The model under review builds one solid part; all positions refer to its coordinate system, in mm. A direction names the side the tool comes from. Round coordinates to 2 decimals unless told otherwise and drop trailing zeros. Loops run counter-clockwise (first coordinate to the right, second up) from the corner with the lowest first, then second, coordinate; pieces in that order, holes last. Notation, with made-up numbers: (83.25, 59.5) -> (126.25, 59.5) arc R9 ccw to (126.25, 69.5) -> close; hole circle Ø8 at (-30, -28). An arc over 180 degrees is marked (long way). Write each question's results on one line, items separated by ' | '. Start each with the question number.
Item 1: Tool access review of faces 1 (the cylindrical face through (16, -2, 0)), 2 (the cylindrical face through (16.93, 5.635, 5.679)), 3 (the cylindrical face through (9, -1.08, -4.88)), 4 (the cylindrical face through (166, -6, 0)), 5 (the cylindrical face through (150.257, 2.731, 1.111)): name each direction out of +Z, -Z, +X, -X, +Y, -Y from which nothing blocks a thin tool from reaching the whole face with its end or side.
Item 2: Clearance check with flat-ended pins moving along their axes: pin 1 Ø3 at (x, y) = (160, 0) entering from -Z; pin 2 Ø3 at (x, y) = (90, -1.5) entering from +Z; pin 3 Ø2 at (x, y) = (106.5, -2) entering from -Z; pin 4 Ø7 at (x, y) = (166.5, -1.5) entering from -Z. State where each tip first meets the part, or that it passes through.
Item 3: Mouldability with a two-part tool opening along X and no side actions: class faces 6 (the flat face through (156.5, -0.1, 4)), 7 (the cylindrical face through (17.38, 3.97, 1.97)) as pulls with the +X half, pulls with the -X half, needs draft (parallel to the pull), parting line crosses it, or undercut.
Item 4: We need section A-A (x = 45). Give the boundary of the cut face in (y, z).
Item 5: For L1, parallel to Z at x = 152, y = 1.5; L2, parallel to X at y = 2.75, z = 4.5; L3, parallel to X at y = -0.25, z = -1.75, list the stretches that pass through material, from the lowest coordinate up. Write a range as from..to.
Autodesk Inventor part; units mm, degrees
ref_plane "FDT_FRONT_XY" through (12, 0, 0) normal (1, 0, 0) x (0, 0, -1)
ref_plane "FDT_FRONT_YZ" through (12, 0, 0) normal (0, 0, -1) x (0, 1, 0)
ref_plane "FDT_FRONT_ZX" through (12, 0, 0) normal (0, 1, 0) x (1, 0, 0)
sketch "Sketch_1" plane through (0, 0, 0) normal (0, 0, 1) x (1, 0, 0)
  line L0 (12, 0) -> (0, 0)
  line L1 (0, 0) -> (0, 5.15)
  line L2 (0, 5.15) -> (0.85, 6)
  line L3 (0.85, 6) -> (7.35, 6)
  line L4 (7.35, 6) -> (8.1743, 5.1757)
  arc A0 (8.1743, 5.1757) -> (8.5985, 5) centre (8.5985, 5.6) ccw
  line L5 (8.5985, 5) -> (9.4, 5)
  arc A1 (9.4, 5) -> (10, 5.6) centre (9.4, 5.6) ccw
  line L6 (10, 5.6) -> (10, 6)
  line L7 (10, 6) -> (12, 6)
  line L8 (12, 6) -> (12, 0)
  line L9 (12, 0) -> (0, 0)
revolve "Revolution1" add sketch "Sketch_1" angle 360 about axis through (12, 0, 0) along (1, 0, 0)
thread "Thread1"
sketch "Sketch_2" plane through (12, 0, 0) normal (1, 0, 0) x (0, 0, -1)
  arc A0 (-7, -3.873) -> (-3.873, -7) centre (0, 0) ccw
  line L0 (-3.873, -7) -> (3.873, -7)
  arc A1 (3.873, -7) -> (7, -3.873) centre (0, 0) ccw
  line L1 (7, -3.873) -> (7, 3.873)
  arc A2 (7, 3.873) -> (3.873, 7) centre (0, 0) ccw
  line L2 (3.873, 7) -> (-3.873, 7)
  arc A3 (-3.873, 7) -> (-7, 3.873) centre (0, 0) ccw
  line L3 (-7, 3.873) -> (-7, -3.873)
extrude "Extrusion1" add sketch "Sketch_2" along normal blind 10
sketch "Sketch_3" plane through (0, 0, 0) normal (0, 0, 1) x (1, 0, 0)
  line L0 (148, 0) -> (22, 0)
  line L1 (22, 0) -> (22, 4.65)
  line L2 (22, 4.65) -> (148, 4.65)
  line L3 (148, 4.65) -> (148, 0)
  line L4 (148, 0) -> (22, 0)
revolve "Revolution2" add sketch "Sketch_3" angle 360 about axis through (148, 0, 0) along (1, 0, 0)
sketch "Sketch_16" plane through (148, 0, 0) normal (1, 0, 0) x (0, 0, -1)
  line L0 (-7, -7) -> (7, -7)
  line L1 (7, -7) -> (7, 7)
  line L2 (7, 7) -> (-7, 7)
  line L3 (-7, 7) -> (-7, -7)
extrude "Extrusion2" add sketch "Sketch_16" along normal blind 10
sketch "Sketch_124" plane through (0, 0, 0) normal (0, 0, 1) x (1, 0, 0)
  line L0 (158, 0) -> (148, 0)
  line L1 (148, 18) -> (148, 8)
  line L2 (148, 8) -> (158, 8)
  line L3 (158, 8) -> (158, 18)
  line L4 (158, 18) -> (148, 18)
revolve "Revolution3" cut sketch "Sketch_124" angle 360 about axis through (158, 0, 0) along (1, 0, 0)
sketch "Sketch_23" plane through (0, 0, 0) normal (0, 0, 1) x (1, 0, 0)
  line L0 (170, 0) -> (158, 0)
  line L1 (158, 0) -> (158, 6)
  line L2 (158, 6) -> (160, 6)
  line L3 (160, 6) -> (160, 5.6)
  arc A0 (160, 5.6) -> (160.6, 5) centre (160.6, 5.6) ccw
  line L4 (160.6, 5) -> (161.4015, 5)
  arc A1 (161.4015, 5) -> (161.8257, 5.1757) centre (161.4015, 5.6) ccw
  line L5 (161.8257, 5.1757) -> (162.65, 6)
  line L6 (162.65, 6) -> (169.15, 6)
  line L7 (169.15, 6) -> (170, 5.15)
  line L8 (170, 5.15) -> (170, 0)
  line L9 (170, 0) -> (158, 0)
revolve "Revolution4" add sketch "Sketch_23" angle 360 about axis through (170, 0, 0) along (1, 0, 0)
thread "Thread2"
sketch "Sketch_6" plane through (0, 0, 0) normal (0, 1, 0) x (-1, 0, 0)
  line L0 (-154, -12) -> (-154, -4)
  line L1 (-154, -4) -> (-170, -4)
  line L2 (-170, -4) -> (-170, 4)
  line L3 (-170, 4) -> (-154, 4)
  line L4 (-154, 4) -> (-154, 12)
  line L5 (-154, 12) -> (-178, 12)
  line L6 (-178, 12) -> (-178, -12)
  line L7 (-178, -12) -> (-154, -12)
extrude "Extrusion3" cut sketch "Sketch_6" along normal mid plane 16
sketch "Sketch_147" plane through (160, 0, 0) normal (1, 0, 0) x (0, 0, -1)
  line L0 (4, 0) -> (-4.2, 0)
  line L1 (-4.2, 0) -> (-4.2, 3.1928)
  line L2 (-4.2, 3.1928) -> (-3, 2.5)
  line L3 (-3, 2.5) -> (-3.5, 2.5)
  line L4 (-3.5, 2.5) -> (-4, 2.2113)
  line L5 (-4, 2.2113) -> (-4, 2)
  line L6 (-4, 2) -> (4, 2)
  line L7 (4, 2) -> (4, 2.2113)
  line L8 (4, 2.2113) -> (3.5, 2.5)
  line L9 (3.5, 2.5) -> (3, 2.5)
  line L10 (3, 2.5) -> (4.2, 3.1928)
  line L11 (4.2, 3.1928) -> (4.2, 0)
  line L12 (4.2, 0) -> (-4.2, 0)
revolve "Revolution5" cut sketch "Sketch_147" angle 360 about axis through (160, 0, -4) along (0, 0, -1)
sketch "Sketch9" plane through (12, 7, 3.873) normal (0, 1, 0) x (1, 0, 0)
  point P0 (6, 3.873)
hole "Hole1" at (18, 7, 0) direction (0, -1, 0) diameter 4.134 depth 7 countersink diameter 5 countersink angle 90
sketch "Sketch10" plane through (148, 7, 3.873) normal (0, 1, 0) x (1, 0, 0)
  point P0 (4, 3.873)
hole "Hole2" at (152, 7, 0) direction (0, -1, 0) diameter 4.134 depth 8 tip angle 120 countersink diameter 5 countersink angle 90
sketch "Sketch_64" plane through (0, 0, 0) normal (0, 0, 1) x (1, 0, 0)
  line L0 (133.5, 0) -> (-4, 0)
  line L1 (-4, 0) -> (-4, 2)
  line L2 (-4, 2) -> (31.5, 2)
  line L3 (31.5, 2) -> (31.5, 4)
  line L4 (31.5, 4) -> (133.5, 4)
  line L5 (133.5, 4) -> (133.5, 0)
  line L6 (133.5, 0) -> (-4, 0)
revolve "Revolution6" cut sketch "Sketch_64" angle 360 about axis through (133.5, 0, 0) along (1, 0, 0)
ref_plane "FDT_FRONT_XY" through (12, 0, 0) normal (1, 0, 0) x (0, 0, -1)
ref_plane "FDT_FRONT_YZ" through (12, 0, 0) normal (0, 0, -1) x (0, 1, 0)
ref_plane "FDT_FRONT_ZX" through (12, 0, 0) normal (0, 1, 0) x (1, 0, 0)
ref_plane "FDT_QSFRONT_XY" through (18, 7, 0) normal (0, 1, 0) x (0, 0, 1)
ref_plane "FDT_QSFRONT_YZ" through (18, 7, 0) normal (0, 0, 1) x (1, 0, 0)
ref_plane "FDT_QSFRONT_ZX" through (18, 7, 0) normal (1, 0, 0) x (0, 1, 0)
ref_plane "FDT_QSREAR_XY" through (152, 7, 0) normal (0, 1, 0) x (0, 0, 1)
ref_plane "FDT_QSREAR_YZ" through (152, 7, 0) normal (0, 0, 1) x (1, 0, 0)
ref_plane "FDT_QSREAR_ZX" through (152, 7, 0) normal (1, 0, 0) x (0, 1, 0)
ref_plane "FDT_REAR_XY" through (158, 0, 0) normal (-1, 0, 0) x (0, 0, -1)
ref_plane "FDT_REAR_YZ" through (158, 0, 0) normal (0, 0, -1) x (0, -1, 0)
ref_plane "FDT_REAR_ZX" through (158, 0, 0) normal (0, -1, 0) x (-1, 0, 0)
ref_plane "FDT_SMBR1_XY" through (31.5, 0, 0) normal (-1, 0, 0) x (0, 0, 1)
ref_plane "FDT_SMBR1_YZ" through (31.5, 0, 0) normal (0, 0, 1) x (0, 1, 0)
ref_plane "FDT_SMBR1_ZX" through (31.5, 0, 0) normal (0, 1, 0) x (-1, 0, 0)
ref_plane "FDT_SMBR2_XY" through (138.5, 0, 0) normal (-1, 0, 0) x (0, 0, 1)
ref_plane "FDT_SMBR2_YZ" through (138.5, 0, 0) normal (0, 0, 1) x (0, 1, 0)
ref_plane "FDT_SMBR2_ZX" through (138.5, 0, 0) normal (0, 1, 0) x (-1, 0, 0)
ref_plane "FDT_SWIVELAXIS_XY" through (160, 0, 0) normal (0, 0, 1) x (1, 0, 0)
ref_plane "FDT_SWIVELAXIS_YZ" through (160, 0, 0) normal (1, 0, 0) x (0, 1, 0)
ref_plane "FDT_SWIVELAXIS_ZX" through (160, 0, 0) normal (0, 1, 0) x (0, 0, 1)
ref_plane "NUT_XY" through (6, 0, 0) normal (1, 0, 0) x (0, 0, -1)
ref_plane "NUT_YZ" through (6, 0, 0) normal (0, 0, -1) x (0, 1, 0)
ref_plane "NUT_ZX" through (6, 0, 0) normal (0, 1, 0) x (1, 0, 0)
ref_plane "ZR_XY" through (0, 0, 0) normal (-1, 0, 0) x (0, 0, -1)
ref_plane "ZR_YZ" through (0, 0, 0) normal (0, 0, -1) x (0, -1, 0)
ref_plane "ZR_ZX" through (0, 0, 0) normal (0, -1, 0) x (-1, 0, 0)
ref_plane "ZYL_XY" through (12, 0, 0) normal (1, 0, 0) x (0, 0, -1)
ref_plane "ZYL_YZ" through (12, 0, 0) normal (0, 0, -1) x (0, 1, 0)
ref_plane "ZYL_ZX" through (12, 0, 0) normal (0, 1, 0) x (1, 0, 0)
properties part number "19182 DSNU-8-100-P---(A----0-ZR)"
Here are the results:
1) face 1: -X | face 2: +Z, +X, -X, +Y | face 3: none | face 4: +X, -Y | face 5: +Y
2) pin 1: passes through | pin 2: stops at z = 4.65 | pin 3: stops at z = -4.54 | pin 4: stops at z = -4
3) face 6: needs draft | face 7: undercut
4) outline: circle Ø9.3 at (0, 0); hole circle Ø8 at (0, 0)
5) L1: z = -7..-2.07, 2.07..7 | L2: x = 0.12..8.08, 9.9..22, 148..154 | L3: x = 133.5..150.9, 153.1..158.02, 161.98..170
